Check sheet for the modelled part. Datum: model origin and axes. Units: mm. Round coordinates to 2 decimals unless told otherwise and drop trailing zeros. Write each loop counter-clockwise with the first axis right and the second up, starting at its lowest first coordinate (ties: lowest second). Pieces come first, ordered by that corner, then holes. Notation, with made-up numbers: M -6,26 L 50,26 A12 ccw 50,39 Z; hole C 82,22 d11. An arc over 180 degrees is marked long. One line per item, written item: value.
from build123d import *

# Parameters (mm, degrees)
SKETCH1_R             = 16
BOSS_EXTRUDE1_DEPTH   = 3
F_3_0MM_DOWEL_HOLE1_D = 3.9
SKETCH6_R             = 3.175
CUT_EXTRUDE3_DEPTH    = 23.825424421
SKETCH14_R            = 1
CUT_EXTRUDE4_DEPTH    = 40
SKETCH7_R             = 1
CUT_EXTRUDE1_DEPTH    = 10.5
SKETCH11_R            = 1.9
CUT_EXTRUDE2_DEPTH    = 2


with BuildPart() as part:
    # Sketch1 → Boss-Extrude1 (new body)
    with BuildSketch(Plane(origin=(0, 0, 0), x_dir=(1, 0, 0), z_dir=(0, 1, 0))):
        with Locations(Location((0, 0, 0), (0, 0, 270))):
            Circle(SKETCH1_R)
    extrude(amount=BOSS_EXTRUDE1_DEPTH)

    # Ø3.0mm Dowel Hole1 (through all)
    with Locations(Plane(origin=(8.485281374, 3, 8.485281374), x_dir=(0, 0, 1), z_dir=(0, 1, 0))):
        with Locations((0, 0), (0, -16.970562748), (-16.970562748, -16.970562748), (-16.970562748, 0)):
            Hole(F_3_0MM_DOWEL_HOLE1_D / 2)

    # Sketch6 → Cut-Extrude3 (cut, through all)
    with BuildSketch(Plane.XZ):
        with Locations(Location((0, 0, 0), (0, 0, 270))):
            Circle(SKETCH6_R)
    extrude(amount=-CUT_EXTRUDE3_DEPTH, mode=Mode.SUBTRACT)

    # Sketch14 → Cut-Extrude4 (cut)
    with BuildSketch(Plane.XY.offset(16)):
        with Locations((0, 1.5)):
            Circle(SKETCH14_R)
    extrude(amount=-CUT_EXTRUDE4_DEPTH, mode=Mode.SUBTRACT)

    # Sketch7 → Cut-Extrude1 (cut)
    with BuildSketch(Plane.XY):
        with Locations((0, -5)):
            Circle(SKETCH7_R)
    extrude(amount=CUT_EXTRUDE1_DEPTH, mode=Mode.SUBTRACT)

    # Sketch11 → Cut-Extrude2 (cut)
    with BuildSketch(Plane.XY.offset(7)):
        with Locations((0, -5)):
            Circle(SKETCH11_R)
    extrude(amount=-CUT_EXTRUDE2_DEPTH, mode=Mode.SUBTRACT)


solid = part.part
Q1. Sectioned sample at D-D on z = 8. Enter the section's corners in (x, y), and give its area (3 significant figures).
Completed:
outline: M -13.86,0 L -10.37,0 L -10.37,3 L -13.86,3 Z; M -6.6,0 L 6.6,0 L 6.6,3 L -6.6,3 Z; M 10.37,0 L 13.86,0 L 13.86,3 L 10.37,3 Z; hole C 0,1.5 d2
area: 57.3 mm^2
Q2. Scan lines: line 1 (X direction, y = 1.8, z = 0) (3 decimals); line 2 (X direction, y = 1.5, z = 9.75); line 3 (Y direction, x = 0, z = 7.25). Record each from-to range of solid material in increasing order. Write a range as [from, to].
Completed:
line 1: [-16, -3.175], [3.175, 16]
line 2: [-12.69, -9.97], [-7, -1], [1, 7], [9.97, 12.69]
line 3: [0, 0.5], [2.5, 3]
Q3. Draft check along Z on faces 1 (the cylindrical face through (-0.217, 0.524, 9.598)), 2 (the cylindrical face through (-6.13, 1.48, 14.78)), 3 (the cylindrical face through (-1.22, 1.48, -2.93)). Enter one of: pulls with the +Z half, pulls with the -Z half, needs draft (parallel to the pull), parting line crosses it, or undercut.
Completed:
face 1: needs draft
face 2: parting line crosses it
face 3: undercut
Q4. Sectioned sample at B-B on z = 0. Enter the section's corners in (x, y) (3 decimals).
Completed:
outline: M -16,0 L -3.175,0 L -3.175,3 L -16,3 Z; M 3.175,0 L 16,0 L 16,3 L 3.175,3 Z
Q5. Depth check by flat-ended pin: P1, Ø1, axis at x = -9, z = -9, coming from the +Y side. Enter the tip coordinate at first touch or a pass-through.
Completed:
P1: through
Q6. Sectioned sample at C-C on y = 1.5. Enter the section's corners in (x, z) (3 decimals).
Completed:
outline: M -1,-15.969 L -1,-3.013 A3.175 cw -1,3.013 L -1,15.969 A16 ccw Z; M 1,-15.969 A16 ccw 1,15.969 L 1,3.013 A3.175 cw 1,-3.013 Z; hole C -8.485,-8.485 d3.9; hole C -8.485,8.485 d3.9; hole C 8.485,-8.485 d3.9; hole C 8.485,8.485 d3.9
Q7. Sectioned sample at A-A on x = 0. Enter the section's corners in (y, z) (3 decimals), and give its area (4 significant figures).
Completed:
outline: M 0,-16 L 0.5,-16 L 0.5,-3.175 L 0,-3.175 Z; M 0,3.175 L 0.5,3.175 L 0.5,16 L 0,16 Z; M 2.5,-16 L 3,-16 L 3,-3.175 L 2.5,-3.175 Z; M 2.5,3.175 L 3,3.175 L 3,16 L 2.5,16 Z
area: 25.65 mm^2
